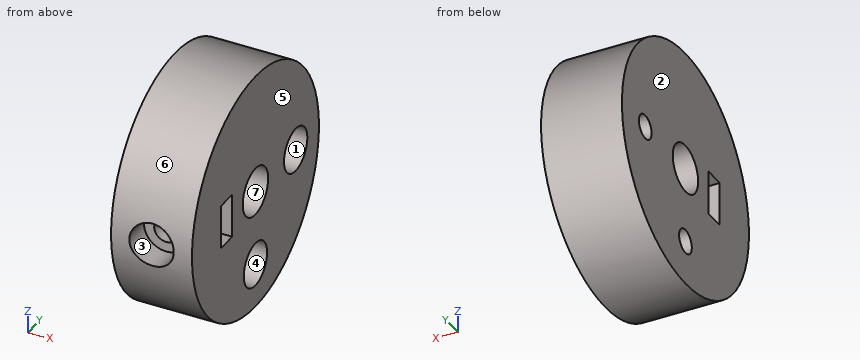
```python
from build123d import *

# Parameters (mm, degrees)
CROQUIS2_R              = 15
CROQUIS2_R_2            = 3
SALIENTE_EXTRUIR1_DEPTH = 10
CROQUIS3_R              = 1.5
CORTAR_EXTRUIR1_DEPTH   = 24.452078799
CROQUIS6_W              = 5.5
CROQUIS6_H              = 2.6
CORTAR_EXTRUIR2_DEPTH   = 24.452078988
CORTAR_EXTRUIR3_START   = -11.5
CROQUIS7_R              = 2.75
CORTAR_EXTRUIR3_DEPTH   = 12.952078988
CROQUIS9_R              = 1.5
CORTAR_EXTRUIR4_DEPTH   = 24.45207897
CORTAR_EXTRUIR5_START   = -2
CROQUIS11_R             = 2.75
CORTAR_EXTRUIR5_DEPTH   = 22.45207897


with BuildPart() as part:
    # Croquis2 → Saliente-Extruir1 (new body)
    with BuildSketch(Plane(origin=(0, 0, 0), x_dir=(0, 0, -1), z_dir=(1, 0, 0))):
        Circle(CROQUIS2_R)
        Circle(CROQUIS2_R_2, mode=Mode.SUBTRACT)
    extrude(amount=-SALIENTE_EXTRUIR1_DEPTH)

    # Croquis3 → Cortar-Extruir1 (cut, through all)
    with BuildSketch(Plane(origin=(0, 0, 0), x_dir=(1, 0, 0), z_dir=(0, 1, 0))):
        with Locations(Location((-5, 0, 0), (0, 0, 270))):
            Circle(CROQUIS3_R)
    extrude(amount=-CORTAR_EXTRUIR1_DEPTH, mode=Mode.SUBTRACT)

    # Croquis6 → Cortar-Extruir2 (cut, through all)
    with BuildSketch(Plane(origin=(0, 0, 0), x_dir=(0, 0, -1), z_dir=(1, 0, 0))):
        with Locations((0, -6.8)):
            Rectangle(CROQUIS6_W, CROQUIS6_H)
    extrude(amount=-CORTAR_EXTRUIR2_DEPTH, mode=Mode.SUBTRACT)

    # Croquis7 → Cortar-Extruir3 (cut, through all)
    with BuildSketch(Plane(origin=(0, 0, 0), x_dir=(1, 0, 0), z_dir=(0, 1, 0)).offset(CORTAR_EXTRUIR3_START)):
        with Locations(Location((-5, 0, 0), (0, 0, 270))):
            Circle(CROQUIS7_R)
    extrude(amount=-CORTAR_EXTRUIR3_DEPTH, mode=Mode.SUBTRACT)

    # Croquis9 → Cortar-Extruir4 (cut, through all)
    with BuildSketch(Plane(origin=(0, 0, 0), x_dir=(0, 0, -1), z_dir=(1, 0, 0))):
        with Locations((9.5, 0)):
            Circle(CROQUIS9_R)
    cortar_extruir4 = extrude(amount=-CORTAR_EXTRUIR4_DEPTH, mode=Mode.SUBTRACT)

    # Croquis11 → Cortar-Extruir5 (cut, through all)
    with BuildSketch(Plane.ZY.offset(10).offset(CORTAR_EXTRUIR5_START)):
        with Locations((-9.5, 0)):
            Circle(CROQUIS11_R)
    cortar_extruir5 = extrude(amount=-CORTAR_EXTRUIR5_DEPTH, mode=Mode.SUBTRACT)

    # Simetr_a1: Cortar-Extruir4, Cortar-Extruir5 across plane
    add(cortar_extruir4.mirror(Plane(origin=(0, 0, 0), x_dir=(0, -0.7071067811865489, 0.7071067811865462), z_dir=(0, 0.7071067811865464, 0.7071067811865488))), mode=Mode.SUBTRACT)
    add(cortar_extruir5.mirror(Plane(origin=(0, 0, 0), x_dir=(0, -0.7071067811865489, 0.7071067811865462), z_dir=(0, 0.7071067811865464, 0.7071067811865488))), mode=Mode.SUBTRACT)


solid = part.part
```
Could you check a few things on this model? Use its own coordinates, in mm. Face numbers are marked on the shaded views. A direction names the side the tool comes from. Give positions to 0.01 mm unless a question says otherwise; leave off trailing zeros. Write each loop counter-clockwise with the first axis right and the second up, starting at its lowest first coordinate (ties: lowest second). Pieces come first, ordered by that corner, then holes. Notation, with made-up numbers: (67, 76.5) - (106, 76.5) arc R10 cw to (106, 95.5) - close; hole circle Ø5 at (6, 10). An arc over 180 degrees is marked (long way). One line per item, written item: value. Start each with the question number.
Item 1: Imagine slicing it at A-A, the plane y = 0. List the corners of the cut face in (x, z) for me, and give its area (3 significant figures).
Item 2: Imagine slicing it at B-B, the plane z = 0. Give the number of separate pieces and of enclosed holes in the cut face, and give its area (3 significant figures).
Item 3: If we mould it in two halves opening along Y, with no side actions, what happens to the marked faces 4, 5, 6 and 7? For each: +Y half, -Y half, draft (parallel to the pull), parting line (faces both ways), or undercut.
Item 4: Please list where these lines run through material, in increasing order: line 1 (Y direction, x = -3.75, z = 2); line 2 (Z direction, x = -0.75, y = 1); line 3 (Z direction, x = -4.5, y = -2). Write a range as from..to.
Item 5: I'm going to push flat-ended pins straight in: pin 1 (6.5 mm diameter, centred on y = 0, z = -9.5, fed in from +X); pin 2 (5.5 mm diameter, centred on y = 0, z = 0, fed in from +X); pin 3 (5 mm diameter, centred on x = -4, z = -8, fed in from +Y); pin 4 (4 mm diameter, centred on x = -3.5, z = 7, fed in from +Y). Where does each tip first touch, or does it pass through?
Item 6: Which directions (+Z, -Z, +X, -X, +Y, -Y) give clear straight access to the entire face, cutting with the end or side of a thin tool? Please do the marked faces 1, 2 and 3.
Item 7: Imagine slicing it at D-D, the plane y = 9.5. List the corners of the cut face in (x, z) for me.
Item 8: Imagine slicing it at C-C, the plane x = -8.5. List the corners of the cut face in (y, z) for me, and give its area (3 significant figures).
Geometry says:
1. outline: (-10, -15) - (0, -15) - (0, -12.25) - (-8, -12.25) - (-8, -11) - (-10, -11) - close; (-10, -8) - (-8, -8) - (-8, -6.75) - (0, -6.75) - (0, -3) - (-10, -3) - close; (-10, 3) - (0, 3) - (0, 15) - (-10, 15) - close
1. area: 190 mm^2
2. separate pieces: 6
2. enclosed holes: 0
2. area: 127 mm^2
3. face 4: undercut
3. face 5: draft
3. face 6: parting line
3. face 7: undercut
4. line 1: -11.5..-8.1, -5.5..-2.24, 2.24..7.61, 11.39..14.87
4. line 2: -14.97..-12.06, -6.94..-2.83, 2.83..14.97
4. line 3: -14.87..-11.39, -7.61..-2.24, 2.24..14.87
5. pin 1: x = 0
5. pin 2: through
5. pin 3: y = 13.96
5. pin 4: y = 14.14
6. face 1: +X
6. face 2: +Z, -Z, -X, +Y, -Y
6. face 3: -Y
7. outline: (-10, -11.61) - (0, -11.61) - (0, -2.75) - (-8, -2.75) - (-8, -1.5) - (-10, -1.5) - close; (-10, 1.5) - (-8, 1.5) - (-8, 2.75) - (0, 2.75) - (0, 11.61) - (-10, 11.61) - close
8. outline: circle Ø30 at (0, 0); hole (-8.1, -2.75) - (-5.5, -2.75) - (-5.5, 2.75) - (-8.1, 2.75) - close; hole circle Ø6 at (0, 0); hole circle Ø3 at (0, -9.5); hole circle Ø3 at (9.5, 0)
8. area: 650 mm^2
